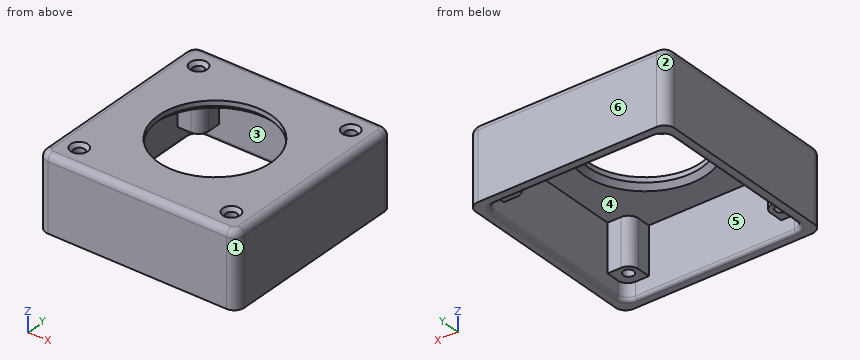
```python
from build123d import *

# Parameters (mm, degrees)
PAD_DEPTH       = 3
SKETCH001_R     = 17
POCKET_DEPTH    = 3.001
PAD001_DEPTH    = 19.3
FILLET_R        = 1
FILLET001_R     = 2
CHAMFER_SIZE    = 1.5
SKETCH003_R     = 1.6
POCKET001_DEPTH = 5
SKETCH004_R     = 1.6
PAD002_DEPTH    = 14.3
CHAMFER001_SIZE = 1


with BuildPart() as part:
    # Sketch → Pad (new body)
    with BuildSketch(Plane.XY):
        with BuildLine():
            Line((-30, 27), (-30, -27))
            ThreePointArc((-30, -27), (-29.12132, -29.12132), (-27, -30))
            Line((-27, -30), (27, -30))
            ThreePointArc((27, -30), (29.12132, -29.12132), (30, -27))
            Line((30, -27), (30, 27))
            ThreePointArc((30, 27), (29.12132, 29.12132), (27, 30))
            Line((27, 30), (-27, 30))
            ThreePointArc((-27, 30), (-29.12132, 29.12132), (-30, 27))
        make_face()
    extrude(amount=PAD_DEPTH)

    # Sketch001 (on Face9 of Pad) → Pocket (cut, through all)
    with BuildSketch(Plane(origin=(0, 0, 0), x_dir=(1, 0, 0), z_dir=(0, 0, -1))):
        Circle(SKETCH001_R)
    extrude(amount=-POCKET_DEPTH, mode=Mode.SUBTRACT)

    # Sketch002 (on Face4 of Pocket) → Pad001 (join)
    with BuildSketch(Plane(origin=(0, 0, 0), x_dir=(1, 0, 0), z_dir=(0, 0, -1))):
        with BuildLine():
            Line((-30, 27), (-30, -27))
            ThreePointArc((-30, -27), (-29.12132, -29.12132), (-27, -30))
            Line((-27, -30), (27, -30))
            ThreePointArc((27, -30), (29.12132, -29.12132), (30, -27))
            Line((30, -27), (30, 27))
            ThreePointArc((30, 27), (29.12132, 29.12132), (27, 30))
            Line((27, 30), (-27, 30))
            ThreePointArc((-27, 30), (-29.12132, 29.12132), (-30, 27))
        make_face()
        with BuildLine():
            Line((-27, 24), (-27, -24))
            ThreePointArc((-27, -24), (-26.12132, -26.12132), (-24, -27))
            Line((-24, -27), (24, -27))
            ThreePointArc((24, -27), (26.12132, -26.12132), (27, -24))
            Line((27, -24), (27, 24))
            ThreePointArc((27, 24), (26.12132, 26.12132), (24, 27))
            Line((24, 27), (-24, 27))
            ThreePointArc((-24, 27), (-26.12132, 26.12132), (-27, 24))
        make_face(mode=Mode.SUBTRACT)
    extrude(amount=PAD001_DEPTH)

    # Fillet
    fillet_edges = [part.edges().sort_by_distance(p)[0] for p in [
        (-27, 0, -19.3),
        (27, 0, -19.3),
        (0, -27, -19.3),
        (0, 27, -19.3),
    ]]
    fillet(fillet_edges, radius=FILLET_R)

    # Fillet001
    fillet001_edges = [part.edges().sort_by_distance(p)[0] for p in [
        (0, 30, 3),
        (-30, 0, 3),
        (0, -30, 3),
        (30, 0, 3),
    ]]
    fillet(fillet001_edges, radius=FILLET001_R)

    # Chamfer
    chamfer_edges = [part.edges().sort_by_distance(p)[0] for p in [
        (-17, 0, 0),
    ]]
    chamfer(chamfer_edges, length=CHAMFER_SIZE)

    # Sketch003 (on Face4 of Chamfer) → Pocket001 (cut)
    with BuildSketch(Plane(origin=(0, 0, 0), x_dir=(1, 0, 0), z_dir=(0, 0, -1))):
        with Locations((-23, 23)):
            Circle(SKETCH003_R)
        with Locations((-23, -23)):
            Circle(SKETCH003_R)
        with Locations((23, -23)):
            Circle(SKETCH003_R)
        with Locations((23, 23)):
            Circle(SKETCH003_R)
    extrude(amount=-POCKET001_DEPTH, mode=Mode.SUBTRACT)

    # Sketch004 (on Face4 of Pocket001) → Pad002 (join)
    with BuildSketch(Plane(origin=(0, 0, 0), x_dir=(1, 0, 0), z_dir=(0, 0, -1))):
        with BuildLine():
            Line((-27, 24), (-27, 20))
            Line((-27, 20), (-23, 20))
            ThreePointArc((-23, 20), (-20.87868, 20.87868), (-20, 23))
            Line((-20, 23), (-20, 27))
            Line((-20, 27), (-24, 27))
            ThreePointArc((-24, 27), (-26.12132, 26.12132), (-27, 24))
        make_face()
        with Locations((-23, 23)):
            Circle(SKETCH004_R, mode=Mode.SUBTRACT)
        with BuildLine():
            Line((23, 20), (27, 20))
            Line((27, 20), (27, 24))
            ThreePointArc((27, 24), (26.12132, 26.12132), (24, 27))
            Line((24, 27), (20, 27))
            Line((20, 27), (20, 23))
            ThreePointArc((20, 23), (20.87868, 20.87868), (23, 20))
        make_face()
        with Locations((23, 23)):
            Circle(SKETCH004_R, mode=Mode.SUBTRACT)
        with BuildLine():
            Line((-23, -20), (-27, -20))
            Line((-27, -20), (-27, -24))
            ThreePointArc((-27, -24), (-26.12132, -26.12132), (-24, -27))
            Line((-24, -27), (-20, -27))
            Line((-20, -27), (-20, -23))
            ThreePointArc((-20, -23), (-20.87868, -20.87868), (-23, -20))
        make_face()
        with Locations((-23, -23)):
            Circle(SKETCH004_R, mode=Mode.SUBTRACT)
        with BuildLine():
            Line((27, -20), (23, -20))
            ThreePointArc((23, -20), (20.87868, -20.87868), (20, -23))
            Line((20, -23), (20, -27))
            Line((20, -27), (24, -27))
            ThreePointArc((24, -27), (26.12132, -26.12132), (27, -24))
            Line((27, -24), (27, -20))
        make_face()
        with Locations((23, -23)):
            Circle(SKETCH004_R, mode=Mode.SUBTRACT)
    extrude(amount=PAD002_DEPTH)

    # Chamfer001
    chamfer001_edges = [part.edges().sort_by_distance(p)[0] for p in [
        (-24.6, -23, 3),
        (21.4, -23, 3),
        (-24.6, 23, 3),
        (21.4, 23, 3),
    ]]
    chamfer(chamfer001_edges, length=CHAMFER001_SIZE)


solid = part.part
```
Here's how the part is built. I have some questions about the finished solid (model axes, mm). Face numbers are marked on the shaded views. A direction names the side the tool comes from. Round coordinates to 2 decimals unless told otherwise and drop trailing zeros. Write each loop counter-clockwise with the first axis right and the second up, starting at its lowest first coordinate (ties: lowest second). Pieces come first, ordered by that corner, then holes. Notation, with made-up numbers: M 89,24 L 108,24 A23 ccw 108,42 Z; hole C -35,-30.75 d4. An arc over 180 degrees is marked long. Answer as CSV lines item,"result". Start each with the question number.
1. I'm going to push flat-ended pins straight in: pin 1 Ø3.5 at (x, y) = (-23, 23) entering from +Z; pin 2 Ø16 at (x, y) = (-4, -9.5) entering from -Z; pin 3 Ø3.5 at (x, y) = (22.5, -25) entering from -Z. Where does each tip first touch, or does it pass through?
2. Suppose I cut it at A-A on y = 0. Write out the boundary of the cut face in (x, z).
3. Thinking about a two-plate mould opening in Y: for the marked faces 1, 2, 3 and 4, which applies, released by +Y, released by -Y, zero draft, split by the parting line, or undercut?
4. Suppose I cut it at C-C on z = -4.5. Write out the boundary of the cut face in (x, y), then the cut area to 3 significant figures.
5. I need wall thicknesses on probe 1 along X at (y, z) = (23, 1.05); probe 2 along X at (y, z) = (-23, -5). Which ranges of each line are inside material? Lowest first, please.
6. On a 3-axis mill with a long thin cutter (end or side, diameter ignored), from which of +Z, -Z, +X, -X, +Y, -Y can I reach the whole of each face in a straight line? I mean the marked faces 5 and 6. Say none if no direction works.
Check result:
1,pin 1,"stops at z = 2.15"
1,pin 2,"stops at z = 0.19"
1,pin 3,"stops at z = -14.3"
2,outline,"M -30,-19.3 L -28,-19.3 A1 ccw -27,-18.3 L -27,0 L -18.5,0 L -17,1.5 L -17,3 L -28,3 A2 ccw -30,1 Z; M 17,1.5 L 18.5,0 L 27,0 L 27,-18.3 A1 ccw 28,-19.3 L 30,-19.3 L 30,1 A2 ccw 28,3 L 17,3 Z"
3,face 1,"released by -Y"
3,face 2,"released by +Y"
3,face 3,"undercut"
3,face 4,"undercut"
4,outline,"M -30,-27 A3 ccw -27,-30 L 27,-30 A3 ccw 30,-27 L 30,27 A3 ccw 27,30 L -27,30 A3 ccw -30,27 Z; hole M -27,-20 L -23,-20 A3 cw -20,-23 L -20,-27 L 20,-27 L 20,-23 A3 cw 23,-20 L 27,-20 L 27,20 L 23,20 A3 cw 20,23 L 20,27 L -20,27 L -20,23 A3 cw -23,20 L -27,20 Z; hole C -23,-23 d3.2; hole C -23,23 d3.2; hole C 23,-23 d3.2; hole C 23,23 d3.2"
4,area,"832 mm2"
5,probe 1,"x = -30 to -24.6, -21.4 to 21.4, 24.6 to 30"
5,probe 2,"x = -30 to -24.6, -21.4 to -20, 20 to 21.4, 24.6 to 30"
6,face 5,"-Z"
6,face 6,"+Z, -Z, +X, -X, +Y"
